Read the model definition and answer for the solid it produces. Units are mm, in the model's axes. Coordinates: 2 decimals unless noted, no trailing zeros. Write each loop counter-clockwise with the first axis right and the second up, starting at its lowest first coordinate (ties: lowest second). Pieces come first, ordered by that corner, then holes. Notation, with made-up numbers: (-37, 88.25) -> (11, 88.25) arc R15 ccw to (11, 94.25) -> close; hole circle Ø8 at (-14.75, 58.25). An arc over 180 degrees is marked (long way). Answer as a JSON object with one key per item and string values. Group by question number.
(1) Find section A-A (z = -124.5). Give the vertices of the cut face in (x, y).
(2) Find section B-B (x = -139). Give the vertices of the cut face in (y, z), then the cut area to 3 significant figures.
(3) Find section C-C (y = 4.7). Give the vertices of the cut face in (x, z).
(4) For a pull along Z with two mould halves and no side action, classify faces 1 (the face through (-203, 0, -343)), 2 (the face through (-140.114, 2.958, -82.108)), 3 (the face through (-192.1, 2.96, -332.73)) as +Z half, -Z half, draft (parallel to the pull), parting line (faces both ways), or undercut.
(5) Flat-ended cylindrical pins translate along their axes: P1, Ø3, axis at x = -343.5, y = 1, coming from the -Z side; P2, Ø1, axis at y = 2.5, z = -359.5, coming from the -X side. Find the tip coordinate at first contact, or state that the pin passes through.
(6) Straight lines are drawn through the part: L1, parallel to X at y = 4.7, z = -392.5; L2, parallel to Z at x = -503, y = 2.7; L3, parallel to X at y = 2.9, z = -293.5. For each, find the intervals that lie inside material, in ascending order.
from build123d import *

# Parameters (mm, degrees)
BOSS_EXTRUDE1_DEPTH = 6


with BuildPart() as part:
    # Sketch1 → Boss-Extrude1 (new body)
    with BuildSketch(Plane(origin=(0, 0, 0), x_dir=(1, 0, 0), z_dir=(0, 1, 0))):
        with BuildLine():
            ThreePointArc((-76.2, 131.982271537), (-131.982271537, 76.2), (-152.4, 0))
            Line((-152.4, 0), (-609.6, 0))
            ThreePointArc((-609.6, 0), (-527.929086147, 304.8), (-304.8, 527.929086147))
            Line((-304.8, 527.929086147), (-76.2, 131.982271537))
        make_face()
        with BuildLine():
            ThreePointArc((-599.516605275, 10), (-578.516992176, 157.601553812), (-521.750777563, 295.459449184))
            ThreePointArc((-521.750777563, 295.459449184), (-519.268832109, 299.8), (-516.750777563, 304.119703222))
            ThreePointArc((-516.750777563, 304.119703222), (-425.745445365, 422.209634839), (-308.418556675, 514.196610158))
            Line((-308.418556675, 514.196610158), (-176.260254038, 285.291715349))
            Line((-176.260254038, 285.291715349), (-171.260254038, 276.631461311))
            Line((-171.260254038, 276.631461311), (-89.706166951, 135.375638912))
            ThreePointArc((-89.706166951, 135.375638912), (-140.642525575, 81.2), (-162.091825827, 10))
            Line((-162.091825827, 10), (-325.2, 10))
            Line((-325.2, 10), (-335.2, 10))
            Line((-335.2, 10), (-599.516605275, 10))
        make_face(mode=Mode.SUBTRACT)
    extrude(amount=BOSS_EXTRUDE1_DEPTH)


solid = part.part
Results below:
{
 "1": {"outline": "(-596.75, 0) -> (-586.53, 0) -> (-586.53, 6) -> (-596.75, 6) -> close; (-104.28, 0) -> (-87.89, 0) -> (-87.89, 6) -> (-104.28, 6) -> close"},
 "2": {"outline": "(0, -240.76) -> (6, -240.76) -> (6, -220.76) -> (0, -220.76) -> close; (0, -83.98) -> (6, -83.98) -> (6, -62.49) -> (0, -62.49) -> close", "area": "249 mm2"},
 "3": {"outline": "(-609.6, 0) arc R609.6 ccw to (-304.8, -527.93) -> (-76.2, -131.98) arc R152.4 cw to (-152.4, 0) -> close; hole (-599.52, -10) arc R599.6 ccw to (-521.75, -295.46) arc R599.6 ccw to (-516.75, -304.12) arc R599.6 ccw to (-308.42, -514.2) -> (-89.71, -135.38) arc R162.4 cw to (-162.09, -10) -> close"},
 "4": {"face 1": "draft", "face 2": "undercut", "face 3": "-Z half"},
 "5": {"P1": "stops at z = -504.63", "P2": "stops at x = -492.68"},
 "6": {"L1": "x = -466.43 to -453.28, -238.16 to -226.61", "L2": "z = -344.39 to -326.36, -10 to 0", "L3": "x = -534.29 to -522.86, -181 to -169.45"}
}
